The model under review builds one solid part; all positions refer to its coordinate system, in mm. Face numbers are marked on the shaded views. A direction names the side the tool comes from. Give positions to 0.01 mm unless a question says otherwise; leave off trailing zeros. Write each loop counter-clockwise with the first axis right and the second up, starting at its lowest first coordinate (ties: lowest second). Pieces come first, ordered by that corner, then holes. Notation, with made-up numbers: M -9,-33.5 L 43,-33.5 A27 ccw 43,-2.5 Z; hole C 77,43.25 d6. An arc over 180 degrees is marked long. Write item = value, one per line. Start each with the question number.
```python
from build123d import *

# Parameters (mm, degrees)
BOSS_EXTRUDE1_DEPTH = 4.7625
SKETCH2_R           = 1.1303
BOSS_EXTRUDE2_DEPTH = 6.858
SKETCH3_R           = 1.143
CUT_EXTRUDE1_DEPTH  = 2.54


with BuildPart() as part:
    # Sketch1 → Boss-Extrude1 (new body)
    with BuildSketch(Plane.XY):
        Polygon((0, 2.749630657), (-2.38125, 1.374815329), (-2.38125, -1.374815329), (0, -2.749630657), (2.38125, -1.374815329), (2.38125, 1.374815329), align=None)
    extrude(amount=BOSS_EXTRUDE1_DEPTH)

    # Sketch2 → Boss-Extrude2 (add)
    with BuildSketch(Plane(origin=(0, 0, 0), x_dir=(-1, 0, 0), z_dir=(0, 0, -1))):
        with Locations(Location((0, 0, 0), (0, 0, 180))):
            Circle(SKETCH2_R)
    extrude(amount=BOSS_EXTRUDE2_DEPTH)

    # Sketch3 → Cut-Extrude1 (cut)
    with BuildSketch(Plane.XY.offset(4.7625)):
        Circle(SKETCH3_R)
    extrude(amount=-CUT_EXTRUDE1_DEPTH, mode=Mode.SUBTRACT)


solid = part.part
```
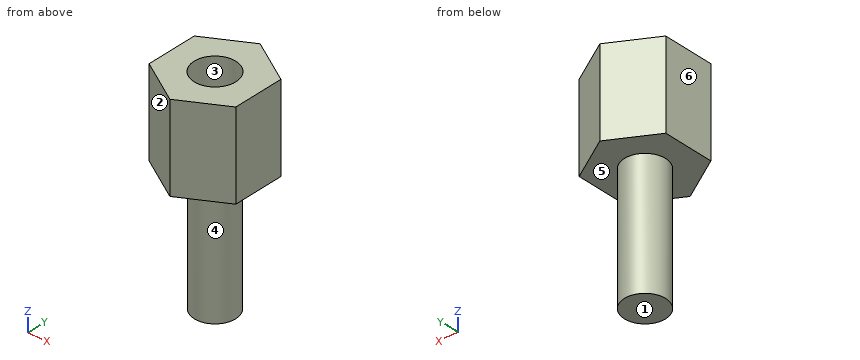
Item 1: We need section A-A, the plane x = 0.45. Write out the cut boundary in (y, z).
Item 2: Clearance check with flat-ended pins moving along their axes: P1, Ø1, axis at x = 1.5, y = 0, coming from the -Z side; P2, Ø0.7, axis at x = 0.5, y = 0, coming from the +Z side; P3, Ø1, axis at x = -0.5, z = -3, coming from the +Y side. State where each tip first meets the part, or that it passes through.
Item 3: We need section D-D, the plane z = 2. Write out the cut boundary in (x, y).
Item 4: For the marked faces 5 and 6, list the 3-axis set-ups (+Z, -Z, +X, -X, +Y, -Y) from which the entire face can be reached by the end or side of a thin tool; tool diameter is ignored.
Item 5: We need section C-C, the plane z = -0.5. Write out the cut boundary in (x, y), and give its area (3 significant figures).
Item 6: To check wall thickness, follow probe 1 along X at (y, z) = (-0.7, 2.5); probe 2 along Z at (x, y) = (-0.75, -0.2); probe 3 along Z at (x, y) = (1.4, 0). State the ranges of each line that lie inside material, in increasing order. Write a range as [from, to].
Item 7: We need section B-B, the plane y = 0. Write out the cut boundary in (x, z).
Item 8: The part is to be moulded in two halves that separate along X. For the marked faces 1, 2, 3 and 4, say which applies: released by +X, released by -X, zero draft, split by the parting line, or undercut.
Worked out:
q1.outline = M -2.49,0 L -1.04,0 L -1.04,-6.86 L 1.04,-6.86 L 1.04,0 L 2.49,0 L 2.49,4.76 L 1.05,4.76 L 1.05,2.22 L -1.05,2.22 L -1.05,4.76 L -2.49,4.76 Z
q2.P1 = -6.86
q2.P2 = 2.22
q2.P3 = 1.13
q3.outline = M -2.38,-1.37 L 0,-2.75 L 2.38,-1.37 L 2.38,1.37 L 0,2.75 L -2.38,1.37 Z
q4.face_5 = -Z
q4.face_6 = +Z, -Z, -X, +Y, -Y
q5.outline = C 0,0 d2.26
q5.area = 4.01 mm²
q6.probe_1 = [-2.38, -0.9], [0.9, 2.38]
q6.probe_2 = [-6.86, 2.22]
q6.probe_3 = [0, 4.76]
q7.outline = M -2.38,0 L -1.13,0 L -1.13,-6.86 L 1.13,-6.86 L 1.13,0 L 2.38,0 L 2.38,4.76 L 1.14,4.76 L 1.14,2.22 L -1.14,2.22 L -1.14,4.76 L -2.38,4.76 Z
q8.face_1 = zero draft
q8.face_2 = released by -X
q8.face_3 = undercut
q8.face_4 = split by the parting line
